```python
from build123d import *

# Parameters (mm, degrees)
BOSS_EXTRUDE1_DEPTH = 9
SKETCH2_R           = 1.55
CUT_EXTRUDE1_DEPTH  = 9


with BuildPart() as part:
    # Sketch1 → Boss-Extrude1 (new body)
    with BuildSketch(Plane(origin=(0, 0, 0), x_dir=(1, 0, 0), z_dir=(0, 1, 0))):
        with BuildLine():
            Line((16.4, 5.016223679), (26.4, 5.016223679))
            Line((26.4, 5.016223679), (26.4, 0))
            Line((26.4, 0), (12.15, 0))
            ThreePointArc((12.15, 0), (0, 12.15), (-12.15, 0))
            Line((-12.15, 0), (-26.4, 0))
            Line((-26.4, 0), (-26.4, 5.016223679))
            Line((-26.4, 5.016223679), (-16.4, 5.016223679))
            ThreePointArc((-16.4, 5.016223679), (0, 17.15), (16.4, 5.016223679))
        make_face()
    extrude(amount=BOSS_EXTRUDE1_DEPTH)

    # Sketch2 → Cut-Extrude1 (cut)
    with BuildSketch(Plane(origin=(0, 0, -5.016223679), x_dir=(-1, 0, 0), z_dir=(0, 0, -1))):
        with Locations((-21.4, 4.5)):
            Circle(SKETCH2_R)
    cut_extrude1 = extrude(amount=-CUT_EXTRUDE1_DEPTH, mode=Mode.SUBTRACT)

    # Mirror1: Cut-Extrude1 across plane
    add(cut_extrude1.mirror(Plane(origin=(0, 0, 0), x_dir=(0, 0, 1), z_dir=(1, 0, 0))), mode=Mode.SUBTRACT)


solid = part.part
```
Verification items for the finished model (mm, model axes). A direction names the side the tool comes from. Round coordinates to 2 decimals unless told otherwise and drop trailing zeros. Order: outer loops, then holes, each group sorted by start corner. A loop starts at its lowest first (then second) coordinate and runs counter-clockwise, first axis right, second up. Notation, with made-up numbers: (10.5, 62.5) -> (17.5, 62.5) arc R22 ccw to (17.5, 75.5) -> close; hole circle Ø10 at (-14.75, 85.25). An arc over 180 degrees is marked (long way). Put each result on its own line as item: value. Start each with the question number.
(1) Section check C-C (x = -21.4). Enter the section's corners in (y, z).
(2) Draft check along Y on faces 4 (the face through (-19, 4, 0)), 5 (the face through (0, 9, -13)), 6 (the face through (-19.968, 3.906, -2.543)), 7 (the face through (19.968, 3.906, -2.543)). Enter one of: +Y half, -Y half, draft (parallel to the pull), parting line (faces both ways), or undercut.
(3) Tool access check on faces 1 (the face through (-0.306, 4.437, -17.147)), 2 (the face through (-23, 3, -5.016)), 3 (the face through (20, 3, -5.016)). Record the directions out of +Z, -Z, +X, -X, +Y, -Y that give a thin tool (end or side, any length) a straight path to the whole face; none if there is none.
(4) Section check A-A (y = 4.5). Enter the section's corners in (x, z), then the cut area to 3 significant figures.
(5) Section check B-B (z = -3). Enter the section's corners in (x, y).
(6) Material ranges on line 1 along Y through (x, z) = (21.4, -1.7); line 2 along Z through (x, y) = (0.5, 6.75); line 3 along Z through (x, y) = (16.5, 5.5), recorded low to high.
(7) Depth check by flat-ended pin: pin 1 Ø2 at (y, z) = (3, -10) entering from -X; pin 2 Ø3.5 at (x, y) = (21.4, 4.5) entering from -Z; pin 3 Ø5 at (x, y) = (-10.5, 7.5) entering from -Z. Enter the tip coordinate at first touch or a pass-through.
(8) Section check D-D (y = 8). Enter the section's corners in (x, z).
Completed:
1. outline: (0, -5.02) -> (2.95, -5.02) -> (2.95, 0) -> (0, 0) -> close; (6.05, -5.02) -> (9, -5.02) -> (9, 0) -> (6.05, 0) -> close
2. face 4: draft
2. face 5: +Y half
2. face 6: undercut
2. face 7: undercut
3. face 1: -Z, +Y, -Y
3. face 2: -Z, -X, +Y, -Y
3. face 3: -Z, +X, +Y, -Y
4. outline: (-26.4, -5.02) -> (-22.95, -5.02) -> (-22.95, 0) -> (-26.4, 0) -> close; (-19.85, -5.02) -> (-16.4, -5.02) arc R17.15 ccw to (16.4, -5.02) -> (19.85, -5.02) -> (19.85, 0) -> (12.15, 0) arc R12.15 cw to (-12.15, 0) -> (-19.85, 0) -> close; (22.95, -5.02) -> (26.4, -5.02) -> (26.4, 0) -> (22.95, 0) -> close
4. area: 294 mm2
5. outline: (-26.4, 0) -> (-11.77, 0) -> (-11.77, 9) -> (-26.4, 9) -> close; (11.77, 0) -> (26.4, 0) -> (26.4, 9) -> (11.77, 9) -> close; hole circle Ø3.1 at (-21.4, 4.5); hole circle Ø3.1 at (21.4, 4.5)
6. line 1: y = 0 to 2.95, 6.05 to 9
6. line 2: z = -17.14 to -12.14
6. line 3: z = -5.02 to 0
7. pin 1: stops at x = -14.6
7. pin 2: stops at z = -5.02
7. pin 3: stops at z = -15.17
8. outline: (-26.4, -5.02) -> (-16.4, -5.02) arc R17.15 ccw to (16.4, -5.02) -> (26.4, -5.02) -> (26.4, 0) -> (12.15, 0) arc R12.15 cw to (-12.15, 0) -> (-26.4, 0) -> close
